For this review, take the finished solid that the model builds, in its own axes (mm). Face numbers are marked on the shaded views. Coordinates: 2 decimals unless noted, no trailing zeros. Loops run counter-clockwise (first coordinate to the right, second up) from the corner with the lowest first, then second, coordinate; pieces in that order, holes last. Notation, with made-up numbers: (-35, -20) -> (18, -20) arc R35 ccw to (18, 14) -> close; hole circle Ø10 at (-30.75, 89). An arc over 180 degrees is marked (long way). One line per item, written item: value.
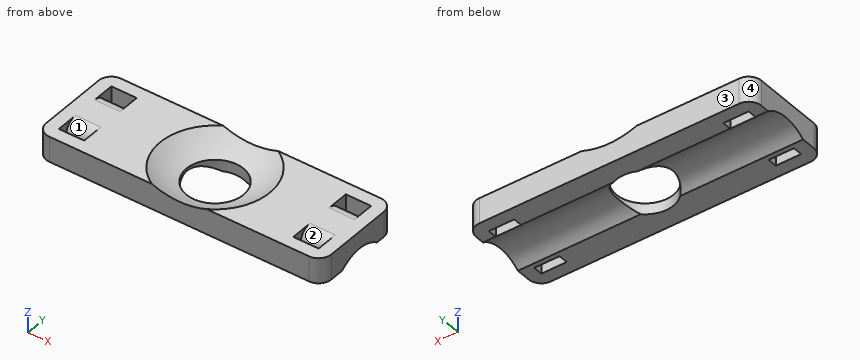
from build123d import *

# Parameters (mm, degrees)
F1_W      = 45
F1_H      = 15
F2_DEPTH  = 4
F6_R      = 4.5
F7_DEPTH  = 16
F8_W      = 4
F8_H      = 1.5
F9_DEPTH  = 25
F10_R     = 2
F11_R     = 2
F13_DEPTH = 50


with BuildPart() as f2:
    # F1 (on Top) → F2 (new body)
    with BuildSketch(Plane.XY):
        Rectangle(F1_W, F1_H)
    extrude(amount=-F2_DEPTH)

    # F4 (on offset) → F5 (revolve, cut)
    with BuildSketch(Plane(origin=(0, 0, 11), x_dir=(1, 0, 0), z_dir=(0, 0, -1))):
        with BuildLine():
            Line((-14, 0), (14, 0))
            ThreePointArc((14, 0), (0, 14), (-14, 0))
        make_face()
    revolve(axis=Axis((0, 0, 11), (1, 0, 0)), mode=Mode.SUBTRACT)

    # F6 (on offset) → F7 (cut)
    with BuildSketch(Plane(origin=(0, 0, 11), x_dir=(1, 0, 0), z_dir=(0, 0, -1))):
        Circle(F6_R)
    extrude(amount=F7_DEPTH, mode=Mode.SUBTRACT)

    # F8 (on face) → F9 (cut)
    with BuildSketch(Plane(origin=(0, 0, -4), x_dir=(1, 0, 0), z_dir=(0, 0, -1))):
        with Locations((-18.5, 4.75)):
            Rectangle(F8_W, F8_H)
        with Locations((18.5, 4.75)):
            Rectangle(F8_W, F8_H)
        with Locations((-18.5, -4.75)):
            Rectangle(F8_W, F8_H)
        with Locations((18.5, -4.75)):
            Rectangle(F8_W, F8_H)
    extrude(amount=-F9_DEPTH, mode=Mode.SUBTRACT)

    # F10
    f10_edges = [f2.edges().sort_by_distance(p)[0] for p in [
        (-18.5, -4, 0),
        (18.5, -4, 0),
        (18.5, 4, 0),
        (-18.5, 4, 0),
    ]]
    fillet(f10_edges, radius=F10_R)

    # F11
    f11_edges = [f2.edges().sort_by_distance(p)[0] for p in [
        (-22.5, -7.5, -2),
        (22.5, -7.5, -2),
        (22.5, 7.5, -2),
        (-22.5, 7.5, -2),
    ]]
    fillet(f11_edges, radius=F11_R)

    # F12 (on face) → F13 (cut)
    with BuildSketch(Plane(origin=(-22.5, 0, 0), x_dir=(0, -1, 0), z_dir=(-1, 0, 0))):
        with BuildLine():
            ThreePointArc((3.2411857887, -4), (-0.4165064602, -2.7009731345), (-4.074198709, -4))
            Line((-4.074198709, -4), (3.2411857887, -4))
        make_face()
    extrude(amount=-F13_DEPTH, mode=Mode.SUBTRACT)


solid = f2.part
1. Take a section at D-D, the plane z = -1.1. Give the boundary of the cut face in (x, y).
Return value:
outline: (-22.5, -5.5) arc R2 ccw to (-20.5, -7.5) -> (20.5, -7.5) arc R2 ccw to (22.5, -5.5) -> (22.5, 5.5) arc R2 ccw to (20.5, 7.5) -> (-20.5, 7.5) arc R2 ccw to (-22.5, 5.5) -> close; hole (-20.5, -5.5) -> (-16.5, -5.5) -> (-16.5, -3.79) -> (-20.5, -3.79) -> close; hole (-20.5, 3.79) -> (-16.5, 3.79) -> (-16.5, 5.5) -> (-20.5, 5.5) -> close; hole circle Ø14.08 at (0, 0); hole (16.5, -5.5) -> (20.5, -5.5) -> (20.5, -3.79) -> (16.5, -3.79) -> close; hole (16.5, 3.79) -> (20.5, 3.79) -> (20.5, 5.5) -> (16.5, 5.5) -> close
2. Insertion check: pin 1 Ø7 at (x, y) = (0, 0) entering from -Z. The pin has a flat end and moves straight along its axis. Give the tip position at first contact, or say it passes through.
Return value:
pin 1: passes through
3. To check wall thickness, follow probe 1 along Y at (x, z) = (0, -3); probe 2 along Y at (x, z) = (4, -2.4); probe 3 along X at (y, z) = (-1, -0.4). State the ranges of each line that lie inside material, in increasing order. Write a range as from..to.
Return value:
probe 1: y = -7.5..-4.5, 4.5..7.5
probe 2: y = -7.5..-2.06, 2.06..7.5
probe 3: x = -22.5..-8.06, 8.06..22.5
4. The part is to be moulded in two halves that separate along X. For the marked faces 1, 2, 3 and 4, say which applies: pulls with the +X half, pulls with the -X half, needs draft (parallel to the pull), parting line crosses it, or undercut.
Return value:
face 1: undercut
face 2: undercut
face 3: needs draft
face 4: pulls with the -X half
5. Take a section at A-A, the plane z = -3.25. Give the number of separate pieces and of enclosed holes in the cut face, and give its area (3 significant figures).
Return value:
separate pieces: 2
enclosed holes: 4
area: 404 mm2
6. Take a section at B-B, the plane y = 1.5. Give the boundary of the cut face in (x, z), and give its area (3 significant figures).
Return value:
outline: (-22.5, -2.8) -> (-4.24, -2.8) -> (-4.24, -2.26) arc R13.92 cw to (-8.53, 0) -> (-22.5, 0) -> close; (4.24, -2.8) -> (22.5, -2.8) -> (22.5, 0) -> (8.53, 0) arc R13.92 cw to (4.24, -2.26) -> close
area: 91.3 mm2
7. Take a section at C-C, the plane x = 1.5. Give the boundary of the cut face in (y, z).
Return value:
outline: (-7.5, -4) -> (-4.24, -4) -> (-4.24, -2.26) arc R13.92 cw to (-7.5, -0.73) -> close; (4.24, -4) -> (7.5, -4) -> (7.5, -0.73) arc R13.92 cw to (4.24, -2.26) -> close
